Input: part model. Units: mm. Frame: model coordinates. Face numbers are marked on the shaded views. A direction names the side the tool comes from. Give positions to 0.01 mm unless a question says otherwise; leave off trailing zeros. Write each loop counter-clockwise with the first axis right and the second up, starting at its lowest first coordinate (ties: lowest second). Pieces come first, ordered by that corner, then holes.
```python
from build123d import *

# Parameters (mm, degrees)
SKETCH1_W               = 14
SKETCH1_H               = 21
SKETCH1_R               = 2.5
SKETCH1_H_2             = 22
BOSS_EXTRUDE1_DEPTH     = 3
BOSS_EXTRUDE6_DEPTH     = 20
CUT_EXTRUDE2_DEPTH      = 95.678403028
CUT_EXTRUDE2_DEPTH_BACK = 95.678403028
SKETCH2_R               = 2.75
CUT_EXTRUDE1_DEPTH      = 5


with BuildPart() as part:
    # Sketch1 → Boss-Extrude1 (new body)
    # profile 1 of 4: a face of its own
    with BuildSketch(Plane(origin=(0, 0, 0), x_dir=(1, 0, 0), z_dir=(0, 1, 0))):
        Polygon((-7, 46), (-7, 40), (7, 40), (7, 19), (-7, 19), (-7, 11), (7, 11), (7, -11), (-7, -11), (-7, -19), (7, -19), (7, -40), (-7, -40), (-7, -46), (7, -46), (10, -46), (10, -40), (10, -18), (10, -12), (10, 12), (10, 18), (10, 40), (10, 46), (7, 46), align=None)
    # profile 2 of 4: a face of its own
    with BuildSketch(Plane(origin=(0, 0, 0), x_dir=(1, 0, 0), z_dir=(0, 1, 0))):
        with Locations((0, -29.5)):
            Rectangle(SKETCH1_W, SKETCH1_H)
        with Locations(Location((0, -30, 0), (0, 0, 270))):
            Circle(SKETCH1_R, mode=Mode.SUBTRACT)
    # profile 3 of 4: a face of its own
    with BuildSketch(Plane(origin=(0, 0, 0), x_dir=(1, 0, 0), z_dir=(0, 1, 0))):
        Rectangle(SKETCH1_W, SKETCH1_H_2)
        with Locations(Location((0, 0, 0), (0, 0, 270))):
            Circle(SKETCH1_R, mode=Mode.SUBTRACT)
    # profile 4 of 4: a face of its own
    with BuildSketch(Plane(origin=(0, 0, 0), x_dir=(1, 0, 0), z_dir=(0, 1, 0))):
        with Locations((0, 29.5)):
            Rectangle(SKETCH1_W, SKETCH1_H)
        with Locations(Location((0, 30, 0), (0, 0, 270))):
            Circle(SKETCH1_R, mode=Mode.SUBTRACT)
    extrude(amount=BOSS_EXTRUDE1_DEPTH)

    # Sketch1_3 → Boss-Extrude6 (add)
    with BuildSketch(Plane(origin=(0, 0, 0), x_dir=(1, 0, 0), z_dir=(0, 1, 0))):
        Polygon((-7, 46), (-7, 40), (7, 40), (7, 19), (-7, 19), (-7, 11), (7, 11), (7, -11), (-7, -11), (-7, -19), (7, -19), (7, -40), (-7, -40), (-7, -46), (7, -46), (10, -46), (10, -40), (10, -18), (10, -12), (10, 12), (10, 18), (10, 40), (10, 46), (7, 46), align=None)
    extrude(amount=BOSS_EXTRUDE6_DEPTH)

    # Sketch3 → Cut-Extrude2 (cut, two sides: drawn at the far end of the back side and taken through both)
    with BuildSketch(Plane.XY.offset(46).offset(-CUT_EXTRUDE2_DEPTH_BACK)):
        Polygon((-7, 20), (-7, 3), (7, 20), align=None)
    extrude(amount=CUT_EXTRUDE2_DEPTH + CUT_EXTRUDE2_DEPTH_BACK, mode=Mode.SUBTRACT)

    # Sketch2 → Cut-Extrude1 (cut)
    with BuildSketch(Plane.ZY.offset(-7)):
        with Locations((-30, 10)):
            Circle(SKETCH2_R)
        with Locations((0, 10)):
            Circle(SKETCH2_R)
        with Locations((30, 10)):
            Circle(SKETCH2_R)
    extrude(amount=-CUT_EXTRUDE1_DEPTH, mode=Mode.SUBTRACT)


solid = part.part
```
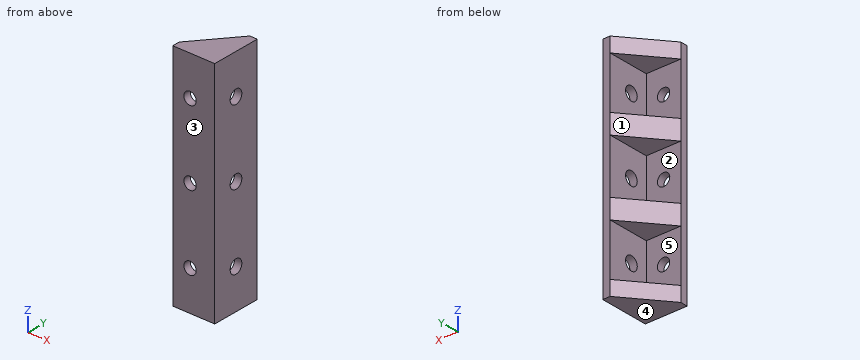
Q1. Section A-A, the plane z = -30. Return the cut outline in (x, y).
Q2. Material intervals for line 1 along Z through (x, y) = (5.25, 17); line 2 along Z through (x, y) = (-1, 2); line 3 along X through (y, z) = (1.9, -30), sorted ascending.
Q3. Mould query, pull axis Z, two halves, no side actions, for the marked faces 3, 4 and 5. Classes: +Z half, -Z half, draft (parallel to the pull), parting line (faces both ways), or undercut.
Q4. Access query for the marked faces 1 and 2. Directions: +Z, -Z, +X, -X, +Y, -Y. A direction counts if a zero-diameter tool reaches every point of the face in a straight line with its end or side. Return the directions, or none.
Q5. Section B-B, the plane x = 0. Return the cut outline in (y, z), then the cut area to 3 significant figures.
Q6. Pin query (flat end, axial travel): pin 1 (5 mm diameter, centred on x = -4.5, y = 12.5, fed in from -Z); pin 2 (7 mm diameter, centred on x = 3, z = -1, fed in from +Y); pin 3 (4 mm diameter, centred on y = 6.5, z = 10.5, fed in from -X); pin 4 (2 mm diameter, centred on y = 6, z = 27, fed in from -X). Return the tip coordinate at first contact, or that it passes through.
Q7. Section C-C, the plane y = 1.75. Return the cut outline in (x, z), then the cut area to 3 significant figures.
Q8. Section D-D, the plane x = 8.75. Return the cut outline in (y, z).
Solutions:
1. outline: (-7, 0) - (-2.5, 0) - (-2.5, 3) - (-7, 3) - close; (2.5, 0) - (10, 0) - (10, 7.25) - (7, 7.25) - (7, 3) - (2.5, 3) - close; (7, 12.75) - (10, 12.75) - (10, 20) - (7, 20) - close
2. line 1: z = -46 to -40, -19 to -11, 11 to 19, 40 to 46
2. line 2: z = -46 to -32.29, -27.71 to -2.29, 2.29 to 27.71, 32.29 to 46
2. line 3: x = -7 to -2.5, 2.5 to 10
3. face 3: draft
3. face 4: -Z half
3. face 5: undercut
4. face 1: +Z, -Z, -X, +Y
4. face 2: -X, +Y
5. outline: (0, -46) - (11.5, -46) - (11.5, -40) - (3, -40) - (3, -32.5) - (0, -32.5) - close; (0, -27.5) - (3, -27.5) - (3, -19) - (11.5, -19) - (11.5, -11) - (3, -11) - (3, -2.5) - (0, -2.5) - close; (0, 2.5) - (3, 2.5) - (3, 11) - (11.5, 11) - (11.5, 19) - (3, 19) - (3, 27.5) - (0, 27.5) - close; (0, 32.5) - (3, 32.5) - (3, 40) - (11.5, 40) - (11.5, 46) - (0, 46) - close
5. area: 469 mm2
6. pin 1: passes through
6. pin 2: stops at y = 3
6. pin 3: stops at x = -5.71
6. pin 4: stops at x = 7
7. outline: (-7, -46) - (10, -46) - (10, 46) - (-7, 46) - close; hole circle Ø5 at (0, -30); hole circle Ø5 at (0, 0); hole circle Ø5 at (0, 30)
7. area: 1,510 mm2
8. outline: (0, -46) - (20, -46) - (20, 46) - (0, 46) - close; hole circle Ø5.5 at (10, -30); hole circle Ø5.5 at (10, 0); hole circle Ø5.5 at (10, 30)
